Build history of the part. All positions in model axes, mm. A direction names the side the tool comes from. Give positions to 0.01 mm unless a question says otherwise; leave off trailing zeros. Loops run counter-clockwise (first coordinate to the right, second up) from the corner with the lowest first, then second, coordinate; pieces in that order, holes last. Notation, with made-up numbers: (-13.5, 45) -> (19.5, 45) arc R22 ccw to (19.5, 71) -> close; hole circle Ø10 at (-27.5, 30.25). An arc over 180 degrees is marked (long way). Answer as a JSON object with one key per item and string values. Group by question number.
Q1. Band-saw the part on C-C, the plane x = 16.5. Write the cut outline in (y, z), plus the area to 3 significant figures.
Q2. Tool access for faces 5 (the flat face through (-16, 9, 1)), 6 (the flat face through (19.1, 0, 5)), 7 (the cylindrical face through (6.25, 11.59, 3.03)): list every direction of +Z, -Z, +X, -X, +Y, -Y with a clear straight run to the whole face (end or side of a thin tool).
Q3. Band-saw the part on A-A, the plane x = 5. Write the cut outline in (y, z).
Q4. Wall check: probe 1 along Y at (x, z) = (-15.6, 2.4); probe 2 along X at (y, z) = (-2.75, 3.25); probe 3 along Y at (x, z) = (0, 4.75). Give the ranges that are in metal, low to high. Write a range as from..to.
Q5. Band-saw the part on D-D, the plane y = -2. Write the cut outline in (x, z), plus the area to 3 significant figures.
Q6. Band-saw the part on B-B, the plane z = 6.5. Write the cut outline in (x, y).
Q7. Drop flat-ended pins along their axis: pin 1 (1.5 mm diameter, centred on x = -16, y = 8.5, fed in from +Z); pin 2 (4 mm diameter, centred on x = -15.6, y = 8.6, fed in from +Z). Give the stop position or say it passes through.
Q8. Two-plate mould, pull along X, no slides. Class faces 1 (the flat face through (13.1, 10, 2)), 2 (the flat face through (-1.5, -11.6, 9.5)), 3 (the flat face through (-19.1, 0, 5)), 4 (the flat face through (-17, 6.1, 2)): pulls with the +X half, pulls with the -X half, needs draft (parallel to the pull), parting line crosses it, or undercut.
from build123d import *

# Parameters (mm, degrees)
F0_W     = 38.2
F0_H     = 24.2
F1_DEPTH = 9.5
F2_T     = -1
F3_R     = 1.5
F4_DEPTH = 2.5
F5_R     = 0.75
F6_DEPTH = 1


with BuildPart() as f1:
    # F0 (on Top) → F1 (new body)
    with BuildSketch(Plane.XY):
        Rectangle(F0_W, F0_H)
    extrude(amount=F1_DEPTH)

    # F2
    f2_openings = [f1.faces().sort_by_distance(p)[0] for p in [
        (0, 0, 9.5),
    ]]
    offset(amount=F2_T, openings=f2_openings)

    # F3 (on face) → F4 (join)
    with BuildSketch(Plane.XY.offset(1)):
        with BuildLine():
            Line((-18.1, 6.1), (-15.6, 6.1))
            ThreePointArc((-15.6, 6.1), (-13.832233, 6.832233), (-13.1, 8.6))
            Line((-13.1, 8.6), (-13.1, 11.1))
            Line((-13.1, 11.1), (-18.1, 11.1))
            Line((-18.1, 11.1), (-18.1, 6.1))
        make_face()
        with Locations((-15.6, 8.6)):
            Circle(F3_R, mode=Mode.SUBTRACT)
        with BuildLine():
            Line((13.1, 11.1), (13.1, 8.6))
            ThreePointArc((13.1, 8.6), (13.832233, 6.832233), (15.6, 6.1))
            Line((15.6, 6.1), (18.1, 6.1))
            Line((18.1, 6.1), (18.1, 11.1))
            Line((18.1, 11.1), (13.1, 11.1))
        make_face()
        with Locations((15.6, 8.6)):
            Circle(F3_R, mode=Mode.SUBTRACT)
    extrude(amount=F4_DEPTH)

    # F5 (on face) → F6 (cut, through all)
    with BuildSketch(Plane.XZ.offset(-11.1)):
        with Locations((5, 3)):
            Circle(F5_R)
        with Locations((7, 3)):
            Circle(F5_R)
    extrude(amount=-F6_DEPTH, mode=Mode.SUBTRACT)


solid = f1.part
Worked answers:
{
 "1": {"outline": "(-12.1, 0) -> (12.1, 0) -> (12.1, 9.5) -> (11.1, 9.5) -> (11.1, 3.5) -> (9.8, 3.5) -> (9.8, 1) -> (7.4, 1) -> (7.4, 3.5) -> (6.1, 3.5) -> (6.1, 1) -> (-11.1, 1) -> (-11.1, 9.5) -> (-12.1, 9.5) -> close", "area": "47.7 mm2"},
 "2": {"face 5": "+Z", "face 6": "+Z, -Z, +X, +Y, -Y", "face 7": "+Y"},
 "3": {"outline": "(-12.1, 0) -> (12.1, 0) -> (12.1, 2.25) -> (11.1, 2.25) -> (11.1, 1) -> (-11.1, 1) -> (-11.1, 9.5) -> (-12.1, 9.5) -> close; (11.1, 3.75) -> (12.1, 3.75) -> (12.1, 9.5) -> (11.1, 9.5) -> close"},
 "4": {"probe 1": "-12.1..-11.1, 6.1..7.1, 10.1..12.1", "probe 2": "-19.1..-18.1, 18.1..19.1", "probe 3": "-12.1..-11.1, 11.1..12.1"},
 "5": {"outline": "(-19.1, 0) -> (19.1, 0) -> (19.1, 9.5) -> (18.1, 9.5) -> (18.1, 1) -> (-18.1, 1) -> (-18.1, 9.5) -> (-19.1, 9.5) -> close", "area": "55.2 mm2"},
 "6": {"outline": "(-19.1, -12.1) -> (19.1, -12.1) -> (19.1, 12.1) -> (-19.1, 12.1) -> close; hole (-18.1, -11.1) -> (18.1, -11.1) -> (18.1, 11.1) -> (-18.1, 11.1) -> close"},
 "7": {"pin 1": "z = 1", "pin 2": "z = 3.5"},
 "8": {"face 1": "undercut", "face 2": "needs draft", "face 3": "pulls with the -X half", "face 4": "undercut"}
}
